Model file for the job. Use its own axes, mm. A direction names the side the tool comes from. Coordinates: 2 decimals unless noted, no trailing zeros. Order: outer loops, then holes, each group sorted by start corner. A loop starts at its lowest first (then second) coordinate and runs counter-clockwise, first axis right, second up.
from build123d import *

# Parameters (mm, degrees)
SKETCH1_R           = 1.5
BOSS_EXTRUDE1_DEPTH = 5
SKETCH2_R           = 3
CUT_EXTRUDE2_DEPTH  = 3.5


with BuildPart() as part:
    # Sketch1 → Boss-Extrude1 (new body)
    with BuildSketch(Plane.XY):
        with BuildLine():
            ThreePointArc((23.501924453, -34.528637882), (39.985677368, -36.01999904), (56.469893836, -34.533770361))
            ThreePointArc((56.469893836, -34.533770361), (65.906534639, -38.094436046), (69.491362273, -47.521924608))
            ThreePointArc((69.491362273, -47.521924608), (68.000001115, -64.005677523), (69.486229793, -80.489893991))
            ThreePointArc((69.486229793, -80.489893991), (65.925564109, -89.926534793), (56.498075547, -93.511362427))
            ThreePointArc((56.498075547, -93.511362427), (40.014322632, -92.02000127), (23.530106164, -93.506229948))
            ThreePointArc((23.530106164, -93.506229948), (14.093465361, -89.945564264), (10.508637727, -80.518075701))
            ThreePointArc((10.508637727, -80.518075701), (11.999998885, -64.034322787), (10.513770207, -47.550106319))
            ThreePointArc((10.513770207, -47.550106319), (14.074435891, -38.113465516), (23.501924453, -34.528637882))
        make_face()
        with Locations((22.755781837, -46.793928993)):
            Circle(SKETCH1_R, mode=Mode.SUBTRACT)
        with Locations((57.226071162, -46.775781992)):
            Circle(SKETCH1_R, mode=Mode.SUBTRACT)
        with Locations((57.244218163, -81.246071317)):
            Circle(SKETCH1_R, mode=Mode.SUBTRACT)
        with Locations((22.773928838, -81.264218317)):
            Circle(SKETCH1_R, mode=Mode.SUBTRACT)
    extrude(amount=BOSS_EXTRUDE1_DEPTH)

    # Sketch2 → Cut-Extrude2 (cut)
    with BuildSketch(Plane.XY.offset(5)):
        with Locations((22.755781837, -46.793928993)):
            Circle(SKETCH2_R)
        with Locations((57.226071162, -46.775781992)):
            Circle(SKETCH2_R)
        with Locations((57.244218163, -81.246071317)):
            Circle(SKETCH2_R)
        with Locations((22.773928838, -81.264218317)):
            Circle(SKETCH2_R)
    extrude(amount=-CUT_EXTRUDE2_DEPTH, mode=Mode.SUBTRACT)


solid = part.part
Q1. Probe line 1 (X direction, y = -47, z = 4.4); line 2 (Y direction, x = 23, z = 3); line 3 (Y direction, x = 22, z = 0.25). List the from-to ranges inside material, lowest first.
Established:
line 1: x = 10.49 to 19.76, 25.75 to 54.23, 60.22 to 69.51
line 2: y = -93.53 to -84.26, -78.27 to -49.78, -43.8 to -34.51
line 3: y = -93.51 to -82.55, -79.98 to -48.09, -45.5 to -34.53
Q2. Which spindle directions (+Z, -Z, +X, -X, +Y, -Y) get a long thin tool onto all of the face, cutting with end or side? Do faces 1 (the face through (56.12, -45.76, 0.74)), 2 (the face through (24.369, -44.264, 3.274)). Say none if no direction does.
Established:
face 1: +Z, -Z
face 2: +Z
Q3. Cut at B-B, the plane z = 2.5. List the corners of the cut face in (x, y), plus the area to 3 significant figures.
Established:
outline: (10.51, -80.52) arc R12.28 ccw to (23.53, -93.51) arc R92 cw to (56.5, -93.51) arc R12.28 ccw to (69.49, -80.49) arc R92 cw to (69.49, -47.52) arc R12.28 ccw to (56.47, -34.53) arc R92 cw to (23.5, -34.53) arc R12.28 ccw to (10.51, -47.55) arc R92 cw to start; hole circle Ø6 at (22.76, -46.79); hole circle Ø6 at (22.77, -81.26); hole circle Ø6 at (57.23, -46.78); hole circle Ø6 at (57.24, -81.25)
area: 3,110 mm2
Q4. Drop flat-ended pins along their axis: P1, Ø1.8, axis at x = 57, y = -46, coming from the +Z side; P2, Ø1.5, axis at x = 34.5, z = 1, coming from the -Y side; P3, Ø3, axis at y = -77.5, z = 2.5, coming from the +X side. Give the stop position or say it passes through.
Established:
P1: stops at z = 1.5
P2: stops at y = -92.23
P3: stops at x = 69.23
Q5. Cut at D-D, the plane x = 33. List the corners of the cut face in (y, z), plus the area to 3 significant figures.
Established:
outline: (-92.29, 0) - (-35.75, 0) - (-35.75, 5) - (-92.29, 5) - close
area: 283 mm2
Q6. Cut at A-A, the plane x = 58. List the corners of the cut face in (y, z).
Established:
outline: (-93.51, 0) - (-82.54, 0) - (-82.54, 1.5) - (-84.15, 1.5) - (-84.15, 5) - (-93.51, 5) - close; (-79.95, 0) - (-48.06, 0) - (-48.06, 1.5) - (-49.67, 1.5) - (-49.67, 5) - (-78.34, 5) - (-78.34, 1.5) - (-79.95, 1.5) - close; (-45.49, 0) - (-34.53, 0) - (-34.53, 5) - (-43.88, 5) - (-43.88, 1.5) - (-45.49, 1.5) - close
Q7. Cut at C-C, the plane y = -49. List the corners of the cut face in (x, z).
Established:
outline: (10.77, 0) - (69.23, 0) - (69.23, 5) - (59.24, 5) - (59.24, 1.5) - (55.21, 1.5) - (55.21, 5) - (24.79, 5) - (24.79, 1.5) - (20.72, 1.5) - (20.72, 5) - (10.77, 5) - close
Q8. Mould opens along X. For faces 3 (the face through (68, -64, 2)), 4 (the face through (56.054, -82.159, 0.74)), 5 (the face through (12, -64, 2)), 6 (the face through (40, -64, 0)) say: pulls with the +X half, pulls with the -X half, needs draft (parallel to the pull), parting line crosses it, or undercut.
Established:
face 3: pulls with the +X half
face 4: undercut
face 5: pulls with the -X half
face 6: needs draft
